from build123d import *

# Parameters (mm, degrees)
BOSS_EXTRU_1_DEPTH       = 5
ESQUISSE2_W              = 5.01
ESQUISSE2_H              = 13.5
ESQUISSE2_W_2            = 23.01
ESQUISSE2_H_2            = 5.01
ENL_V_MAT_EXTRU_7_DEPTH  = 10
ESQUISSE3_R              = 3.05
ENL_V_MAT_EXTRU_8_DEPTH  = 5
ENL_V_MAT_EXTRU_12_DEPTH = 5
ESQUISSE5_R              = 3.05
ESQUISSE5_R_2            = 1.55
ESQUISSE5_R_3            = 1.5
ENL_V_MAT_EXTRU_13_DEPTH = 5
ENL_V_MAT_EXTRU_14_DEPTH = 5


with BuildPart() as part:
    # Esquisse1 → Boss.-Extru.1 (new body)
    with BuildSketch(Plane.XY):
        with BuildLine():
            Line((130, -105), (-130, -105))
            ThreePointArc((-130, -105), (-137.071067812, -102.071067812), (-140, -95))
            Line((-140, -95), (-140, 105))
            Line((-140, 105), (140, 105))
            Line((140, 105), (140, -95))
            ThreePointArc((140, -95), (137.071067812, -102.071067812), (130, -105))
        make_face()
    extrude(amount=BOSS_EXTRU_1_DEPTH)

    # Esquisse2 → Enl_v. mat.-Extru.7 (cut)
    with BuildSketch(Plane.XY.offset(5)):
        with Locations((-36.505, -7.25)):
            Rectangle(ESQUISSE2_W, ESQUISSE2_H)
        with Locations((-36.505, 21.25)):
            Rectangle(ESQUISSE2_W, ESQUISSE2_H)
        with Locations((-36.505, -35.75)):
            Rectangle(ESQUISSE2_W, ESQUISSE2_H)
        with Locations((-61.505, -7.25)):
            Rectangle(ESQUISSE2_W, ESQUISSE2_H)
        with Locations((-61.505, 21.25)):
            Rectangle(ESQUISSE2_W, ESQUISSE2_H)
        with Locations((-61.505, -35.75)):
            Rectangle(ESQUISSE2_W, ESQUISSE2_H)
        with Locations((-82.505, 21.25)):
            Rectangle(ESQUISSE2_W, ESQUISSE2_H)
        with Locations((-82.505, -7.25)):
            Rectangle(ESQUISSE2_W, ESQUISSE2_H)
        with Locations((-82.505, -35.75)):
            Rectangle(ESQUISSE2_W, ESQUISSE2_H)
        with Locations((82.505, 21.25)):
            Rectangle(ESQUISSE2_W, ESQUISSE2_H)
        with Locations((61.505, -54.495)):
            Rectangle(ESQUISSE2_W_2, ESQUISSE2_H_2)
        with Locations((61.505, 40.495)):
            Rectangle(ESQUISSE2_W_2, ESQUISSE2_H_2)
        with Locations((82.505, -35.75)):
            Rectangle(ESQUISSE2_W, ESQUISSE2_H)
        with Locations((82.505, -7.25)):
            Rectangle(ESQUISSE2_W, ESQUISSE2_H)
        with Locations((61.505, -35.75)):
            Rectangle(ESQUISSE2_W, ESQUISSE2_H)
        with Locations((61.505, -7.25)):
            Rectangle(ESQUISSE2_W, ESQUISSE2_H)
        with Locations((61.505, 21.25)):
            Rectangle(ESQUISSE2_W, ESQUISSE2_H)
        with Locations((36.505, -35.75)):
            Rectangle(ESQUISSE2_W, ESQUISSE2_H)
        with Locations((36.505, -7.25)):
            Rectangle(ESQUISSE2_W, ESQUISSE2_H)
        with Locations((-61.505, 40.495)):
            Rectangle(ESQUISSE2_W_2, ESQUISSE2_H_2)
        with Locations((-61.505, -54.495)):
            Rectangle(ESQUISSE2_W_2, ESQUISSE2_H_2)
        with Locations((36.505, 21.25)):
            Rectangle(ESQUISSE2_W, ESQUISSE2_H)
    extrude(amount=-ENL_V_MAT_EXTRU_7_DEPTH, mode=Mode.SUBTRACT)

    # Esquisse3 → Enl_v. mat.-Extru.8 (cut)
    with BuildSketch(Plane.XY.offset(5)):
        with Locations((-126, 36.4987829)):
            Circle(ESQUISSE3_R)
        with Locations((-126, -26.5012171)):
            Circle(ESQUISSE3_R)
        with Locations((-126, 53.4987829)):
            Circle(ESQUISSE3_R)
        with Locations((-126, -56.5012171)):
            Circle(ESQUISSE3_R)
        with Locations((-106, 53.4987829)):
            Circle(ESQUISSE3_R)
        with Locations((-106, -56.5012171)):
            Circle(ESQUISSE3_R)
        with Locations(Location((106, -56.5012171, 0), (0, 0, 180))):
            Circle(ESQUISSE3_R)
        with Locations(Location((106, 53.4987829, 0), (0, 0, 180))):
            Circle(ESQUISSE3_R)
        with Locations(Location((126, -56.5012171, 0), (0, 0, 180))):
            Circle(ESQUISSE3_R)
        with Locations(Location((126, 53.4987829, 0), (0, 0, 180))):
            Circle(ESQUISSE3_R)
        with Locations(Location((126, -26.5012171, 0), (0, 0, 180))):
            Circle(ESQUISSE3_R)
        with Locations(Location((126, 36.4987829, 0), (0, 0, 180))):
            Circle(ESQUISSE3_R)
    extrude(amount=-ENL_V_MAT_EXTRU_8_DEPTH, mode=Mode.SUBTRACT)

    # Esquisse4 → Enl_v. mat.-Extru.12 (cut)
    with BuildSketch(Plane.XY.offset(5)):
        with BuildLine():
            ThreePointArc((110, 105), (102.928932188, 102.071067812), (100, 95))
            Line((100, 95), (100, 68))
            ThreePointArc((100, 68), (99.121320344, 65.878679656), (97, 65))
            Line((97, 65), (-97, 65))
            ThreePointArc((-97, 65), (-99.121320344, 65.878679656), (-100, 68))
            Line((-100, 68), (-100, 95))
            ThreePointArc((-100, 95), (-102.928932188, 102.071067812), (-110, 105))
            Line((-110, 105), (110, 105))
        make_face()
        with BuildLine():
            ThreePointArc((119.5, 19.9987829), (126, 26.4987829), (132.5, 19.9987829))
            Line((132.5, 19.9987829), (132.5, -10.0012171))
            ThreePointArc((132.5, -10.0012171), (126, -16.5012171), (119.5, -10.0012171))
            Line((119.5, -10.0012171), (119.5, 19.9987829))
        make_face()
        with BuildLine():
            Line((-119.5, -10.0012171), (-119.5, 19.9987829))
            ThreePointArc((-119.5, 19.9987829), (-126, 26.4987829), (-132.5, 19.9987829))
            Line((-132.5, 19.9987829), (-132.5, -10.0012171))
            ThreePointArc((-132.5, -10.0012171), (-126, -16.5012171), (-119.5, -10.0012171))
        make_face()
        with BuildLine():
            ThreePointArc((-130, 105), (-137.071067812, 102.071067812), (-140, 95))
            Line((-140, 95), (-140, 105))
            Line((-140, 105), (-130, 105))
        make_face()
        with BuildLine():
            ThreePointArc((130, 105), (137.071067812, 102.071067812), (140, 95))
            Line((140, 95), (140, 105))
            Line((140, 105), (130, 105))
        make_face()
    extrude(amount=-ENL_V_MAT_EXTRU_12_DEPTH, mode=Mode.SUBTRACT)

    # Esquisse5 → Enl_v. mat.-Extru.13 (cut)
    with BuildSketch(Plane.XY.offset(5)):
        with Locations((-100, -90)):
            Circle(ESQUISSE5_R)
        with Locations((-133, -98)):
            Circle(ESQUISSE5_R_2)
        with Locations((-133, 98)):
            Circle(ESQUISSE5_R_2)
        with Locations(Location((133, -98, 0), (0, 0, 180))):
            Circle(ESQUISSE5_R_2)
        with Locations(Location((100, -90, 0), (0, 0, 180))):
            Circle(ESQUISSE5_R)
        with Locations(Location((133, 98, 0), (0, 0, 180))):
            Circle(ESQUISSE5_R_2)
        with Locations((-113, 98)):
            Circle(ESQUISSE5_R_3)
        with Locations(Location((113, 98, 0), (0, 0, 180))):
            Circle(ESQUISSE5_R_3)
        with Locations((-10, -98)):
            Circle(ESQUISSE5_R_3)
        with Locations(Location((10, -98, 0), (0, 0, 180))):
            Circle(ESQUISSE5_R_3)
        with Locations((-20, 58)):
            Circle(ESQUISSE5_R_3)
        with Locations((-10, 58)):
            Circle(ESQUISSE5_R_3)
        with Locations(Location((10, 58, 0), (0, 0, 180))):
            Circle(ESQUISSE5_R_3)
        with Locations(Location((20, 58, 0), (0, 0, 180))):
            Circle(ESQUISSE5_R_3)
        with BuildLine():
            Line((-9.1, 10.1), (9.1, 10.1))
            ThreePointArc((9.1, 10.1), (9.807106781, 9.807106781), (10.1, 9.1))
            Line((10.1, 9.1), (10.1, -9.1))
            ThreePointArc((10.1, -9.1), (9.807106781, -9.807106781), (9.1, -10.1))
            Line((9.1, -10.1), (-9.1, -10.1))
            ThreePointArc((-9.1, -10.1), (-9.807106781, -9.807106781), (-10.1, -9.1))
            Line((-10.1, -9.1), (-10.1, 9.1))
            ThreePointArc((-10.1, 9.1), (-9.807106781, 9.807106781), (-9.1, 10.1))
        make_face()
    extrude(amount=-ENL_V_MAT_EXTRU_13_DEPTH, mode=Mode.SUBTRACT)

    # Esquisse6 → Enl_v. mat.-Extru.14 (cut)
    with BuildSketch(Plane.XY.offset(5)):
        with BuildLine():
            Line((-41.25, -42.75), (-41.25, -47.25))
            ThreePointArc((-41.25, -47.25), (-43, -49), (-44.75, -47.25))
            Line((-44.75, -47.25), (-44.75, -42.75))
            ThreePointArc((-44.75, -42.75), (-43, -41), (-41.25, -42.75))
        make_face()
        with BuildLine():
            Line((-26.25, -42.75), (-26.25, -47.25))
            ThreePointArc((-26.25, -47.25), (-28, -49), (-29.75, -47.25))
            Line((-29.75, -47.25), (-29.75, -42.75))
            ThreePointArc((-29.75, -42.75), (-28, -41), (-26.25, -42.75))
        make_face()
        with BuildLine():
            Line((26.25, -42.75), (26.25, -47.25))
            ThreePointArc((26.25, -47.25), (28, -49), (29.75, -47.25))
            Line((29.75, -47.25), (29.75, -42.75))
            ThreePointArc((29.75, -42.75), (28, -41), (26.25, -42.75))
        make_face()
        with BuildLine():
            Line((41.25, -42.75), (41.25, -47.25))
            ThreePointArc((41.25, -47.25), (43, -49), (44.75, -47.25))
            Line((44.75, -47.25), (44.75, -42.75))
            ThreePointArc((44.75, -42.75), (43, -41), (41.25, -42.75))
        make_face()
    extrude(amount=-ENL_V_MAT_EXTRU_14_DEPTH, mode=Mode.SUBTRACT)


solid = part.part
Check sheet for the modelled part. Datum: model origin and axes. Units: mm. A direction names the side the tool comes from. Give positions to 0.01 mm unless a question says otherwise; leave off trailing zeros. Write each loop counter-clockwise with the first axis right and the second up, starting at its lowest first coordinate (ties: lowest second). Pieces come first, ordered by that corner, then holes. Notation, with made-up numbers: (60.25, 37) -> (94.25, 37) arc R29 cw to (94.25, 73) -> close; hole circle Ø10 at (-5, -0.5). An arc over 180 degrees is marked (long way). One line per item, written item: value. Start each with the question number.
Item 1: Tool access check on faces 4 (the cylindrical face through (125.9, 26.5, 2.5)), 5 (the flat face through (2, -22, 0)), 6 (the cylindrical face through (103.01, 102.15, 2.54)). Record the directions out of +Z, -Z, +X, -X, +Y, -Y that give a thin tool (end or side, any length) a straight path to the whole face; none if there is none.
Item 2: Section check A-A on y = -90. Record the cut outline in (x, z), then the cut area to 3 significant figures.
Item 3: Section check B-B on z = 1.8. State how many separate pieces and enclosed holes the cut face has, then the cut area to 3 significant figures.
Item 4: Gauge pin test, flat ends, axial feed: pin 1 (1.5 mm diameter, centred on x = -87, z = 1.5, fed in from +Y); pin 2 (5.5 mm diameter, centred on x = 126, y = 53.5, fed in from -Z). Record the tip position at first contact, or that the pin passes through.
Item 5: Material ranges on probe 1 along Y at (x, z) = (-53, 1.8); probe 2 along X at (y, z) = (10.5, 2.9); probe 3 along X at (y, z) = (-44, 0.7), recorded low to high. Write a range as from..to.
Item 6: Draft check along Y on faces 1 (the cylindrical face through (-102.85, 101.99, 2.54)), 2 (the flat face through (2, -22, 5)), 3 (the cylindrical face through (-123.183, -27.669, 2.535)). Enter one of: +Y half, -Y half, draft (parallel to the pull), parting line (faces both ways), or undercut.
Results list:
1. face 4: +Z, -Z
1. face 5: -Z, +X, -X, +Y, -Y
1. face 6: +Z, -Z, +Y
2. outline: (-140, 0) -> (-103.05, 0) -> (-103.05, 5) -> (-140, 5) -> close; (-96.95, 0) -> (96.95, 0) -> (96.95, 5) -> (-96.95, 5) -> close; (103.05, 0) -> (140, 0) -> (140, 5) -> (103.05, 5) -> close
2. area: 1,340 mm²
3. separate pieces: 1
3. enclosed holes: 55
3. area: 46,900 mm²
4. pin 1: y = 65
4. pin 2: through
5. probe 1: -105..-57, -51.99..37.99, 43..65
5. probe 2: -140..-132.5, -119.5..119.5, 132.5..140
5. probe 3: -140..-44.75, -41.25..-29.75, -26.25..26.25, 29.75..41.25, 44.75..140
6. face 1: +Y half
6. face 2: draft
6. face 3: undercut
